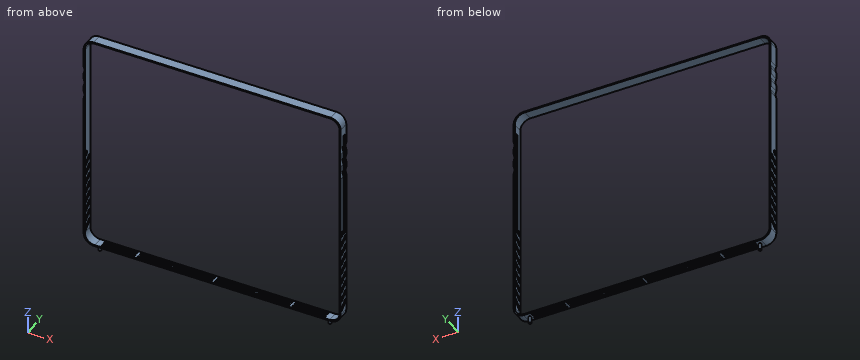
from build123d import *

# Parameters (mm, degrees)
F0_W      = 493.776
F0_H      = 420.624
F1_DEPTH  = 9.8425
F2_R      = 19.05
F3_R      = 19.05
F4_R      = 19.05
F5_R      = 19.05
F7_DEPTH  = 9.8435
F8_DEPTH  = 50.8
F9_DEPTH  = 9.8435
F11_DEPTH = 381
F12_DEPTH = 381
F13_W     = 76.2
F13_H     = 5.08
F13_W_2   = 63.499903
F13_W_3   = 64.816944
F14_DEPTH = 254
F16_DEPTH = 63.5
F17_R     = 2.479907
F18_DEPTH = 223.012
F19_DEPTH = 208.28
F20_W     = 5.08
F20_H     = 203.2
F21_DEPTH = 254


with BuildPart() as f1:
    # F0 (on Front) → F1 (new body, symmetric)
    with BuildSketch(Plane.XZ):
        Rectangle(F0_W, F0_H)
    extrude(amount=F1_DEPTH, both=True)

    # F2
    f2_edges = [f1.edges().sort_by_distance(p)[0] for p in [
        (246.888, 0, 210.312),
    ]]
    fillet(f2_edges, radius=F2_R)

    # F3
    f3_edges = [f1.edges().sort_by_distance(p)[0] for p in [
        (-246.888, 0, 210.312),
    ]]
    fillet(f3_edges, radius=F3_R)

    # F4
    f4_edges = [f1.edges().sort_by_distance(p)[0] for p in [
        (246.888, 0, -210.312),
    ]]
    fillet(f4_edges, radius=F4_R)

    # F5
    f5_edges = [f1.edges().sort_by_distance(p)[0] for p in [
        (-246.888, 0, -210.312),
    ]]
    fillet(f5_edges, radius=F5_R)

    # F6 (on Front) → F7 (cut, through all)
    with BuildSketch(Plane.XZ):
        with BuildLine():
            ThreePointArc((244.856, 189.23), (239.276384, 202.700384), (225.806, 208.28))
            Line((225.806, 208.28), (-225.806, 208.28))
            ThreePointArc((-225.806, 208.28), (-239.276384, 202.700384), (-244.856, 189.23))
            Line((-244.856, 189.23), (-244.856, -189.23))
            ThreePointArc((-244.856, -189.23), (-239.276384, -202.700384), (-225.806, -208.28))
            Line((-225.806, -208.28), (225.806, -208.28))
            ThreePointArc((225.806, -208.28), (239.276384, -202.700384), (244.856, -189.23))
            Line((244.856, -189.23), (244.856, 189.23))
        make_face()
    extrude(amount=-F7_DEPTH, mode=Mode.SUBTRACT)

    # F6 (on Front) → F8 (cut)
    with BuildSketch(Plane.XZ):
        with BuildLine():
            ThreePointArc((244.856, 189.23), (239.276384, 202.700384), (225.806, 208.28))
            Line((225.806, 208.28), (-225.806, 208.28))
            ThreePointArc((-225.806, 208.28), (-239.276384, 202.700384), (-244.856, 189.23))
            Line((-244.856, 189.23), (-244.856, -189.23))
            ThreePointArc((-244.856, -189.23), (-239.276384, -202.700384), (-225.806, -208.28))
            Line((-225.806, -208.28), (225.806, -208.28))
            ThreePointArc((225.806, -208.28), (239.276384, -202.700384), (244.856, -189.23))
            Line((244.856, -189.23), (244.856, 189.23))
        make_face()
    extrude(amount=-F8_DEPTH, mode=Mode.SUBTRACT)

    # F6 (on Front) → F9 (cut, through all)
    with BuildSketch(Plane.XZ):
        with BuildLine():
            ThreePointArc((244.856, 189.23), (239.276384, 202.700384), (225.806, 208.28))
            Line((225.806, 208.28), (-225.806, 208.28))
            ThreePointArc((-225.806, 208.28), (-239.276384, 202.700384), (-244.856, 189.23))
            Line((-244.856, 189.23), (-244.856, -189.23))
            ThreePointArc((-244.856, -189.23), (-239.276384, -202.700384), (-225.806, -208.28))
            Line((-225.806, -208.28), (225.806, -208.28))
            ThreePointArc((225.806, -208.28), (239.276384, -202.700384), (244.856, -189.23))
            Line((244.856, -189.23), (244.856, 189.23))
        make_face()
    extrude(amount=F9_DEPTH, mode=Mode.SUBTRACT)

    # F10 (on Right) → F11 (cut)
    with BuildSketch(Plane.YZ):
        Polygon((7.3025, -40.869898), (7.3025, -34.519898), (-7.3025, -46.578553), (-7.3025, -52.924015), align=None)
        Polygon((7.3025, -59.915363), (7.3025, -53.569898), (-7.3025, -65.624015), (-7.3025, -71.969477), align=None)
        Polygon((-7.3025, -27.542157), (-7.3025, -33.878553), (-1.32043, -27.528553), (-1.32043, -21.173388), align=None)
        Polygon((7.3025, -72.615363), (-7.3025, -84.669477), (-7.3025, -91.024636), (7.3025, -78.324636), align=None)
        Polygon((7.3025, -91.024636), (-7.3025, -103.724636), (-7.3025, -110.074636), (7.3025, -97.374636), align=None)
        Polygon((7.3025, -110.074636), (-7.3025, -122.774636), (-7.3025, -129.124636), (7.3025, -116.424636), align=None)
        Polygon((7.3025, -129.124636), (-7.3025, -141.824636), (-7.3025, -148.174636), (7.3025, -135.474636), align=None)
        Polygon((7.3025, -148.174636), (-7.3025, -160.874636), (-7.3025, -167.224636), (7.3025, -154.524636), align=None)
        Polygon((7.3025, -167.224636), (-7.3025, -179.924636), (-7.3025, -186.274636), (7.3025, -173.574636), align=None)
    extrude(amount=-F11_DEPTH, mode=Mode.SUBTRACT)

    # F10 (on Right) → F12 (cut)
    with BuildSketch(Plane.YZ):
        Polygon((7.3025, -40.869898), (7.3025, -34.519898), (-7.3025, -46.578553), (-7.3025, -52.924015), align=None)
        Polygon((7.3025, -59.915363), (7.3025, -53.569898), (-7.3025, -65.624015), (-7.3025, -71.969477), align=None)
        Polygon((-7.3025, -27.542157), (-7.3025, -33.878553), (-1.32043, -27.528553), (-1.32043, -21.173388), align=None)
        Polygon((7.3025, -72.615363), (-7.3025, -84.669477), (-7.3025, -91.024636), (7.3025, -78.324636), align=None)
        Polygon((7.3025, -91.024636), (-7.3025, -103.724636), (-7.3025, -110.074636), (7.3025, -97.374636), align=None)
        Polygon((7.3025, -110.074636), (-7.3025, -122.774636), (-7.3025, -129.124636), (7.3025, -116.424636), align=None)
        Polygon((7.3025, -129.124636), (-7.3025, -141.824636), (-7.3025, -148.174636), (7.3025, -135.474636), align=None)
        Polygon((7.3025, -148.174636), (-7.3025, -160.874636), (-7.3025, -167.224636), (7.3025, -154.524636), align=None)
        Polygon((7.3025, -167.224636), (-7.3025, -179.924636), (-7.3025, -186.274636), (7.3025, -173.574636), align=None)
    extrude(amount=F12_DEPTH, mode=Mode.SUBTRACT)

    # F13 (on Top) → F14 (cut)
    with BuildSketch(Plane.XY):
        with Locations((-40.64, -4.7625)):
            Rectangle(F13_W, F13_H)
        with Locations((-40.64, 4.7625)):
            Rectangle(F13_W, F13_H)
        Polygon((-215.138, -2.553835), (-215.138, -7.633835), (-151.638097, -7.523006), (-151.638097, -2.553835), align=None)
        with Locations((-183.388048, 4.7625)):
            Rectangle(F13_W_2, F13_H)
        Polygon((-146.125123, -2.553835), (-146.125123, -7.523006), (-81.281083, -7.523006), (-81.308179, -2.2225), align=None)
        with Locations((-113.716651, 4.7625)):
            Rectangle(F13_W_3, F13_H)
        with Locations((40.64, -4.7625)):
            Rectangle(F13_W, F13_H)
        with Locations((40.64, 4.7625)):
            Rectangle(F13_W, F13_H)
        Polygon((81.308179, -2.2225), (81.281083, -7.523006), (146.125123, -7.523006), (146.125123, -2.553835), align=None)
        with Locations((113.716651, 4.7625)):
            Rectangle(F13_W_3, F13_H)
        Polygon((151.638097, -2.553835), (151.638097, -7.523006), (215.138, -7.633835), (215.138, -2.553835), align=None)
        with Locations((183.388048, 4.7625)):
            Rectangle(F13_W_2, F13_H)
    extrude(amount=-F14_DEPTH, mode=Mode.SUBTRACT)

    # F15 (on Front) → F16 (cut, symmetric)
    with BuildSketch(Plane.XZ):
        with BuildLine():
            ThreePointArc((-250.468968, 134.112), (-246.872017, 140.014539), (-245.618, 146.812))
            ThreePointArc((-245.618, 146.812), (-271.465461, 164.607983), (-278.867032, 134.112))
            ThreePointArc((-278.867032, 134.112), (-264.668, 140.462), (-250.468968, 134.112))
        make_face()
        with BuildLine():
            ThreePointArc((-250.468968, 134.112), (-264.668, 127.762), (-278.867032, 134.112))
            ThreePointArc((-278.867032, 134.112), (-283.718, 121.412), (-278.867032, 108.712))
            ThreePointArc((-278.867032, 108.712), (-264.668, 115.062), (-250.468968, 108.712))
            ThreePointArc((-250.468968, 108.712), (-246.872017, 114.614539), (-245.618, 121.412))
            ThreePointArc((-245.618, 121.412), (-246.872017, 128.209461), (-250.468968, 134.112))
        make_face()
        with BuildLine():
            ThreePointArc((-250.468968, 108.712), (-264.668, 102.362), (-278.867032, 108.712))
            ThreePointArc((-278.867032, 108.712), (-271.465461, 78.216017), (-245.618, 96.012))
            ThreePointArc((-245.618, 96.012), (-246.872017, 102.809461), (-250.468968, 108.712))
        make_face()
        with BuildLine():
            ThreePointArc((250.468968, 108.712), (257.870539, 78.216017), (283.718, 96.012))
            ThreePointArc((283.718, 96.012), (282.463983, 102.809461), (278.867032, 108.712))
            ThreePointArc((278.867032, 108.712), (264.668, 102.362), (250.468968, 108.712))
        make_face()
        with BuildLine():
            ThreePointArc((250.468968, 108.712), (264.668, 115.062), (278.867032, 108.712))
            ThreePointArc((278.867032, 108.712), (282.463983, 114.614539), (283.718, 121.412))
            ThreePointArc((283.718, 121.412), (282.463983, 128.209461), (278.867032, 134.112))
            ThreePointArc((278.867032, 134.112), (264.668, 127.762), (250.468968, 134.112))
            ThreePointArc((250.468968, 134.112), (245.618, 121.412), (250.468968, 108.712))
        make_face()
        with BuildLine():
            ThreePointArc((283.718, 146.812), (257.870539, 164.607983), (250.468968, 134.112))
            ThreePointArc((250.468968, 134.112), (264.668, 140.462), (278.867032, 134.112))
            ThreePointArc((278.867032, 134.112), (282.463983, 140.014539), (283.718, 146.812))
        make_face()
    extrude(amount=F16_DEPTH, both=True, mode=Mode.SUBTRACT)

    # F17 (on Top) → F18 (join)
    with BuildSketch(Plane.XY):
        with Locations((-221.302345, 0)):
            Circle(F17_R)
        with Locations((221.302345, 0)):
            Circle(F17_R)
    extrude(amount=-F18_DEPTH)

    # F17 (on Top) → F19 (cut)
    with BuildSketch(Plane.XY):
        with Locations((-221.302345, 0)):
            Circle(F17_R)
        with Locations((221.302345, 0)):
            Circle(F17_R)
    extrude(amount=-F19_DEPTH, mode=Mode.SUBTRACT)

    # F20 (on Right) → F21 (cut)
    with BuildSketch(Plane.YZ):
        with Locations((2.54, 71.648132)):
            Rectangle(F20_W, F20_H)
    extrude(amount=F21_DEPTH, mode=Mode.SUBTRACT)


solid = f1.part
Input: part model. Units: mm. Frame: model coordinates. Round coordinates to 2 decimals unless told otherwise and drop trailing zeros. Write each loop counter-clockwise with the first axis right and the second up, starting at its lowest first coordinate (ties: lowest second). Pieces come first, ordered by that corner, then holes.
1) Cut plane A-A (z = 45). Return the cut outline in (x, y), then the cut area to 3 significant figures.
2) Ray query, L1, parallel to Z at x = 129, y = -7.75; L2, parallel to X at y = -1.5, z = 184; L3, parallel to X at y = 5, z = 190.5. Return the intervals inside material, ascending.
3) Contact query for flat-ended pins moving along their axis: P1, Ø2, axis at y = -4.5, z = 150.5, coming from the +X side; P2, Ø2, axis at y = 4, z = -209.5, coming from the +X side; P3, Ø2, axis at x = 246, y = 3.5, coming from the -Z side. Output: stop coordinate, or through.
4) Cut plane B-B (x = -32). Return the cut outline in (y, z).
5) Cut plane C-C (x = 186.5). Return the cut outline in (y, z).
Geometry says:
1. outline: (-246.89, -9.84) - (-244.86, -9.84) - (-244.86, 9.84) - (-246.89, 9.84) - close; (244.86, -9.84) - (246.89, -9.84) - (246.89, 0) - (244.86, 0) - close; (244.86, 5.08) - (246.89, 5.08) - (246.89, 9.84) - (244.86, 9.84) - close
1. area: 69.7 mm2
2. L1: z = -210.31 to -208.28, 208.28 to 210.31
2. L2: x = -246.89 to -244.86, 244.86 to 246.89
2. L3: x = -246.89 to -244.81, 244.81 to 246.89
3. P1: stops at x = 246.2
3. P2: stops at x = 235.95
3. P3: stops at z = -199.53
4. outline: (-9.84, -210.31) - (-7.3, -210.31) - (-7.3, -208.28) - (-9.84, -208.28) - close; (-9.84, 208.28) - (9.84, 208.28) - (9.84, 210.31) - (-9.84, 210.31) - close; (-2.22, -210.31) - (2.22, -210.31) - (2.22, -208.28) - (-2.22, -208.28) - close; (7.3, -210.31) - (9.84, -210.31) - (9.84, -208.28) - (7.3, -208.28) - close
5. outline: (-9.84, -210.31) - (-7.58, -210.31) - (-7.58, -208.28) - (-9.84, -208.28) - close; (-9.84, 208.28) - (9.84, 208.28) - (9.84, 210.31) - (-9.84, 210.31) - close; (-2.55, -210.31) - (2.22, -210.31) - (2.22, -208.28) - (-2.55, -208.28) - close; (7.3, -210.31) - (9.84, -210.31) - (9.84, -208.28) - (7.3, -208.28) - close
